Check sheet for the modelled part. Datum: model origin and axes. Units: mm. A direction names the side the tool comes from. Give positions to 0.01 mm unless a question says otherwise; leave off trailing zeros. Loops run counter-clockwise (first coordinate to the right, second up) from the corner with the lowest first, then second, coordinate; pieces in that order, holes last. Notation, with made-up numbers: M 48,-36 L 62,-36 A13 cw 62,-23 Z; hole C 48.25,74.5 d11. An arc over 180 degrees is marked long. Write each question's results on one line, items separated by ' | '. Start each with the question number.
1. Sectioned sample at C-C on x = -36. Record the cut outline in (y, z).
2. Tool access check on faces 5 (the flat face through (-10.61, -13, 48)), 6 (the flat face through (24, -13, -4.653)), 7 (the flat face through (50.804, -13, -3)), 8 (the flat face through (30, -13, 40.609)). Record the directions out of +Z, -Z, +X, -X, +Y, -Y that give a thin tool (end or side, any length) a straight path to the whole face; none if there is none.
3. Sectioned sample at B-B on y = -9. Give the number of separate pieces and of enclosed holes in the cut face, and give its area (3 significant figures).
4. Material ranges on line 1 along X through (y, z) = (-4, 16); line 2 along X through (y, z) = (-1, 49.5); line 3 along Z through (x, y) = (-8, -2.5), recorded low to high.
5. Draft check along Z on faces 1 (the flat face through (9.452, -13, 48)), 2 (the flat face through (-25.754, -12.522, -53.812)), 3 (the flat face through (-30, -13, 40.609)), 4 (the flat face through (-1, -13, 40.609)). Enter one of: pulls with the +Z half, pulls with the -Z half, needs draft (parallel to the pull), parting line crosses it, or undercut.
6. Go/stop test with flat-tipped pins: pin 1 (7.5 mm diameter, centred on x = 25.5, y = -10, fed in from +Z); pin 2 (12.5 mm diameter, centred on x = 31, y = -18, fed in from -Z); pin 3 (5.5 mm diameter, centred on y = -15.5, z = 44, fed in from +X). Record where each tip stops, or that it passes through.
7. Sectioned sample at A-A on z = 21.5. Record the cut outline in (x, y).
```python
from build123d import *

# Parameters (mm, degrees)
F0_W     = 39.707024
F0_H     = 29.651739
F0_W_2   = 39.7002
F1_DEPTH = 18.542
F2_DEPTH = 25.4


with BuildPart() as f1:
    # F0 (on Front) → F1 (new body)
    with BuildSketch(Plane.XZ):
        Polygon((-50.795936, 40.608853), (-50.795936, 0), (-50.795936, -46.078143), (0, -61.765383), (50.804064, -46.078143), (50.804064, 0), (50.804064, 40.608853), (9.452418, 40.608853), (4.051034, 40.608853), (-5.18992, 40.608853), (-10.609858, 40.608853), align=None)
        Polygon((-44.896944, -42.148899), (-44.896944, -4.764843), (-5.196902, -4.652967), (-4.745259, -54.160614), align=None, mode=Mode.SUBTRACT)
        Polygon((4.754341, -54.160614), (4.301752, -4.652967), (44.001952, -4.652967), (44.001952, -42.041767), align=None, mode=Mode.SUBTRACT)
        with Locations((-25.043432, 17.793344)):
            Rectangle(F0_W, F0_H, mode=Mode.SUBTRACT)
        with Locations((24.151852, 17.793344)):
            Rectangle(F0_W_2, F0_H, mode=Mode.SUBTRACT)
    extrude(amount=F1_DEPTH)

    # F0 (on Front) → F2 (join)
    with BuildSketch(Plane.XZ):
        Polygon((-50.795936, 40.608853), (-50.795936, 0), (-50.795936, -46.078143), (0, -61.765383), (50.804064, -46.078143), (50.804064, 0), (50.804064, 40.608853), (9.452418, 40.608853), (4.051034, 40.608853), (-5.18992, 40.608853), (-10.609858, 40.608853), align=None)
        Polygon((-44.896944, -42.148899), (-44.896944, -4.764843), (-5.196902, -4.652967), (-4.745259, -54.160614), align=None, mode=Mode.SUBTRACT)
        Polygon((4.754341, -54.160614), (4.301752, -4.652967), (44.001952, -4.652967), (44.001952, -42.041767), align=None, mode=Mode.SUBTRACT)
        with Locations((-25.043432, 17.793344)):
            Rectangle(F0_W, F0_H, mode=Mode.SUBTRACT)
        with Locations((24.151852, 17.793344)):
            Rectangle(F0_W_2, F0_H, mode=Mode.SUBTRACT)
        Polygon((-10.609858, 55.941623), (-10.609858, 40.608853), (-5.18992, 40.608853), (-5.18992, 51.311865), (4.051034, 51.311865), (4.051034, 40.608853), (9.452418, 40.608853), (9.452418, 55.941623), align=None)
    extrude(amount=F2_DEPTH)


solid = f1.part
```
Output values:
1) outline: M -25.4,-50.65 L 0,-50.65 L 0,-44.81 L -25.4,-44.81 Z; M -25.4,-4.74 L 0,-4.74 L 0,2.97 L -25.4,2.97 Z; M -25.4,32.62 L 0,32.62 L 0,40.61 L -25.4,40.61 Z
2) face 5: +Z, -X, +Y, -Y | face 6: +Y, -Y | face 7: +Z, -Z, +X, +Y, -Y | face 8: +Z, +X, +Y, -Y
3) separate pieces: 1 | enclosed holes: 5 | area: 4,010 mm2
4) line 1: -50.8 to -44.9, -5.19 to 4.3, 44 to 50.8 | line 2: -10.61 to -5.19, 4.05 to 9.45 | line 3: -59.29 to -53.19, -4.66 to 2.97, 32.62 to 55.94
5) face 1: needs draft | face 2: pulls with the -Z half | face 3: pulls with the +Z half | face 4: undercut
6) pin 1: z = 40.61 | pin 2: z = -54.12 | pin 3: x = 9.45
7) outline: M -50.8,-25.4 L -44.9,-25.4 L -44.9,0 L -50.8,0 Z; M -5.19,-25.4 L 4.3,-25.4 L 4.3,0 L -5.19,0 Z; M 44,-25.4 L 50.8,-25.4 L 50.8,0 L 44,0 Z
